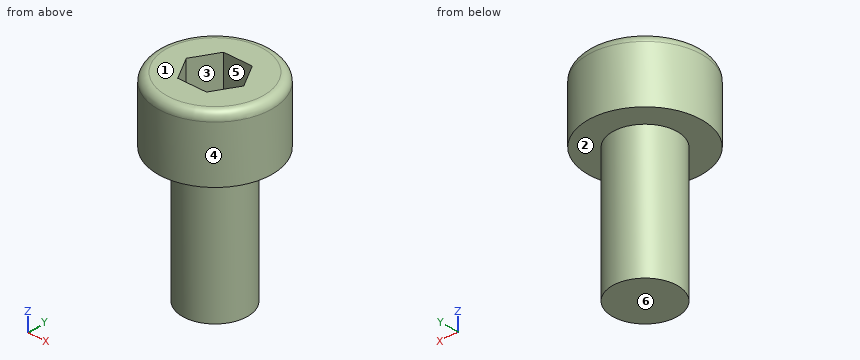
```python
from build123d import *

# Parameters (mm, degrees)
SKETCH1_R           = 3.425
BOSS_EXTRUDE1_DEPTH = 3.9
SKETCH2_R           = 1.95
BOSS_EXTRUDE2_DEPTH = 8
CUT_EXTRUDE1_DEPTH  = 2.5
FILLET1_R           = 0.5


with BuildPart() as part:
    # Sketch1 → Boss-Extrude1 (new body)
    with BuildSketch(Plane.XY):
        Circle(SKETCH1_R)
    extrude(amount=BOSS_EXTRUDE1_DEPTH)

    # Sketch2 → Boss-Extrude2 (add)
    with BuildSketch(Plane(origin=(0, 0, 0), x_dir=(-1, 0, 0), z_dir=(0, 0, -1))):
        Circle(SKETCH2_R)
    extrude(amount=BOSS_EXTRUDE2_DEPTH)

    # Sketch3 → Cut-Extrude1 (cut)
    with BuildSketch(Plane.XY.offset(3.9)):
        Polygon((1.732050808, 0), (0.866025404, 1.5), (-0.866025404, 1.5), (-1.732050808, 0), (-0.866025404, -1.5), (0.866025404, -1.5), align=None)
    extrude(amount=-CUT_EXTRUDE1_DEPTH, mode=Mode.SUBTRACT)

    # Fillet1
    fillet1_edges = [part.edges().sort_by_distance(p)[0] for p in [
        (-3.425, 0, 3.9),
    ]]
    fillet(fillet1_edges, radius=FILLET1_R)


solid = part.part
```
Geometry: final body of the model. Coordinates: model frame, mm. Face numbers are marked on the shaded views. A direction names the side the tool comes from. Coordinates: 2 decimals unless noted, no trailing zeros. Loops run counter-clockwise (first coordinate to the right, second up) from the corner with the lowest first, then second, coordinate; pieces in that order, holes last. Notation, with made-up numbers: (87, -7.5) -> (91, -7.5) arc R31 ccw to (91, 28.5) -> close; hole circle Ø2 at (31.5, 67.5). An arc over 180 degrees is marked (long way). Use a Markdown table: item, result. Add a question column.
(1) Line query: line 1 along Y through (x, z) = (0, -4); line 2 along X through (y, z) = (1.25, -1.75); line 3 along Z through (x, y) = (2.25, -0.5). Output: solid intervals per line, ascending.
(2) Pin query (flat end, axial travel): pin 1 Ø3.5 at (x, y) = (0.5, 0) entering from +Z; pin 2 Ø1.5 at (x, z) = (1, 1) entering from -Y. Return the tip coordinate at first contact, or that it passes through.
(3) Section query A-A, the plane x = 0. Return loops of the section in (y, z) (3 decimals).
(4) Section query B-B, the plane z = -6.5. Return loops of the section in (x, y), plus the area to 3 significant figures.
(5) Access query for the marked faces 1, 2 and 3. Directions: +Z, -Z, +X, -X, +Y, -Y. A direction counts if a zero-diameter tool reaches every point of the face in a straight line with its end or side. Return the directions, or none.
(6) Mould query, pull axis Y, two halves, no side actions, for the marked faces 4, 5 and 6. Classes: pulls with the +Y half, pulls with the -Y half, needs draft (parallel to the pull), parting line crosses it, or undercut.
Answer:
| question | item | result |
|---|---|---|
| 1 | line 1 | y = -1.95 to 1.95 |
| 1 | line 2 | x = -1.5 to 1.5 |
| 1 | line 3 | z = 0 to 3.9 |
| 2 | pin 1 | stops at z = 3.9 |
| 2 | pin 2 | stops at y = -3.42 |
| 3 | outline | (-3.425, 0) -> (-1.95, 0) -> (-1.95, -8) -> (1.95, -8) -> (1.95, 0) -> (3.425, 0) -> (3.425, 3.4) arc R0.5 ccw to (2.925, 3.9) -> (1.5, 3.9) -> (1.5, 1.4) -> (-1.5, 1.4) -> (-1.5, 3.9) -> (-2.925, 3.9) arc R0.5 ccw to (-3.425, 3.4) -> close |
| 4 | outline | circle Ø3.9 at (0, 0) |
| 4 | area | 11.9 mm^2 |
| 5 | face 1 | +Z, +X, -X, +Y, -Y |
| 5 | face 2 | -Z |
| 5 | face 3 | +Z |
| 6 | face 4 | parting line crosses it |
| 6 | face 5 | undercut |
| 6 | face 6 | needs draft |
